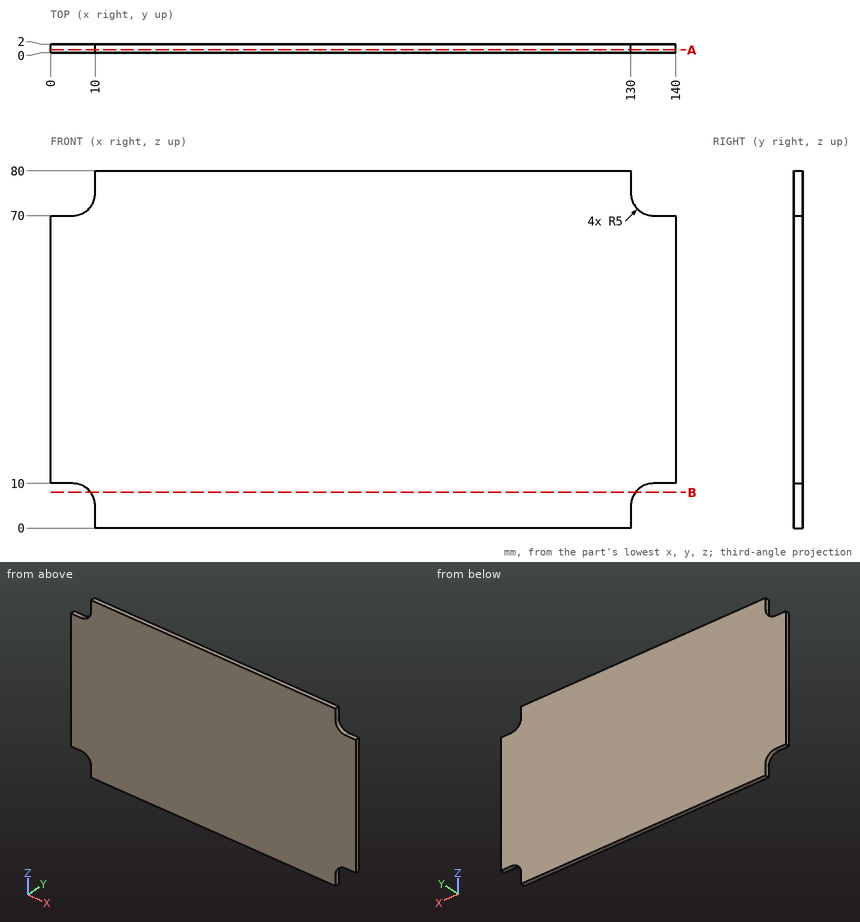
The figure shows three views and two pictorial views of one solid part (mm, origin at its lowest corner). Answer the questions. Round coordinates to 2 decimals unless told otherwise and drop trailing zeros. Loops run counter-clockwise (first coordinate to the right, second up) from the corner with the lowest first, then second, coordinate; pieces in that order, holes last. Notation, with made-up numbers: (22.25, 14) -> (30.25, 14) arc R32 ccw to (30.25, 42) -> close; hole circle Ø7 at (46.5, 72). An arc over 180 degrees is marked (long way). Use one line per item in the form item = value.
(1) Flat-ended cylindrical pins translate along their axes: P1, Ø0.6, axis at x = 138.5, y = 0.5, coming from the +Z side; P2, Ø0.6, axis at y = 1, z = 77.5, coming from the +X side; P3, Ø0.6, axis at y = 0.5, z = 77, coming from the -X side. Find the tip coordinate at first contact, or state that the pin passes through.
Answer list:
P1 = 70
P2 = 130
P3 = 10
(2) Straight lines are drawn through the part: line 1 (Z direction, x = 7.5, y = 1.7); line 2 (X direction, y = 0.5, z = 8). For each, find the intervals that lie inside material, in ascending order.
Answer list:
line_1 = 9.33 to 70.67
line_2 = 9 to 131
(3) Find section B-B on z = 8. Give the vertices of the cut face in (x, y).
Answer list:
outline = (9, 0) -> (131, 0) -> (131, 2) -> (9, 2) -> close
(4) Find section A-A on y = 0.7. Give the vertices of the cut face in (x, z), then the cut area to 3 significant figures.
Answer list:
outline = (0, 10) -> (5, 10) arc R5 cw to (10, 5) -> (10, 0) -> (130, 0) -> (130, 5) arc R5 cw to (135, 10) -> (140, 10) -> (140, 70) -> (135, 70) arc R5 cw to (130, 75) -> (130, 80) -> (10, 80) -> (10, 75) arc R5 cw to (5, 70) -> (0, 70) -> close
area = 10,800 mm2
